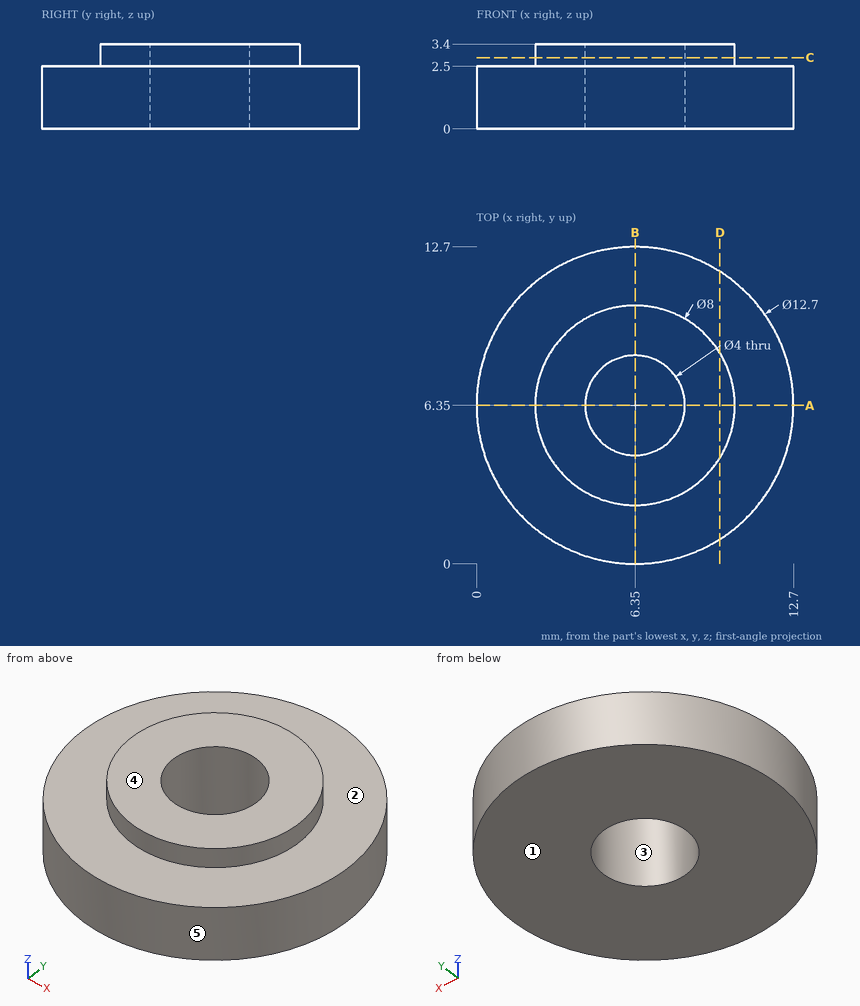
Answer from the drawing. Dimensions are ordinates in mm from the lowest x, y and z of the part. A direction names the side the tool comes from. Coordinates: 2 decimals unless noted, no trailing zeros. Write each loop counter-clockwise with the first axis right and the second up, starting at its lowest first coordinate (ties: lowest second). Pieces come first, ordered by that corner, then holes. Notation, with made-up numbers: M 81.5,82.25 L 133.5,82.25 A19 ccw 133.5,104.25 Z; hole C 87.25,41.5 d10. An arc over 180 degrees is marked long. Put each result on its own line as item: value. Start each with the question number.
1. Flat-ended cylindrical pins translate along their axes: P1, Ø1, axis at y = 11, z = 2.5, coming from the +X side; P2, Ø3, axis at x = 2, y = 2.5, coming from the +Z side; P3, Ø2, axis at x = 11, z = 3, coming from the +Y side. Find the tip coordinate at first contact, or state that the pin passes through.
2. Consider line 1 (Y direction, x = 6.35, z = 1.1); line 2 (Y direction, x = 6.35, z = 2.55); line 3 (Z direction, x = 7.25, y = 10.75). Determine where each line is inside the solid, lowest interval first. Write a range as from..to.
3. For a pull along X with two mould halves and no side action, classify the marked faces 3, 4 and 5 as pulls with the +X half, pulls with the -X half, needs draft (parallel to the pull), parting line crosses it, or undercut.
4. A cutting plane is placed at C-C on z = 2.85. Write down the section's boundary in (x, y), then the cut area to 3 significant figures.
5. A cutting plane is placed at D-D on x = 9.75. Write down the section's boundary in (y, z), then the cut area to 3 significant figures.
6. A cutting plane is placed at A-A on y = 6.35. Write down the section's boundary in (x, z).
7. Which of the six approach directions +Z, -Z, +X, -X, +Y, -Y give full straight-line access (tool end or side, diameter ignored) to the marked faces 1 and 2?
Resolved:
1. P1: stops at x = 11.16
1. P2: stops at z = 2.5
1. P3: stops at y = 11.45
2. line 1: y = 0..4.35, 8.35..12.7
2. line 2: y = 2.35..4.35, 8.35..10.35
2. line 3: z = 0..2.5
3. face 3: undercut
3. face 4: needs draft
3. face 5: parting line crosses it
4. outline: C 6.35,6.35 d8; hole C 6.35,6.35 d4
4. area: 37.7 mm2
5. outline: M 0.99,0 L 11.71,0 L 11.71,2.5 L 8.46,2.5 L 8.46,3.4 L 4.24,3.4 L 4.24,2.5 L 0.99,2.5 Z
5. area: 30.6 mm2
6. outline: M 0,0 L 4.35,0 L 4.35,3.4 L 2.35,3.4 L 2.35,2.5 L 0,2.5 Z; M 8.35,0 L 12.7,0 L 12.7,2.5 L 10.35,2.5 L 10.35,3.4 L 8.35,3.4 Z
7. face 1: -Z, +X, -X, +Y, -Y
7. face 2: +Z
